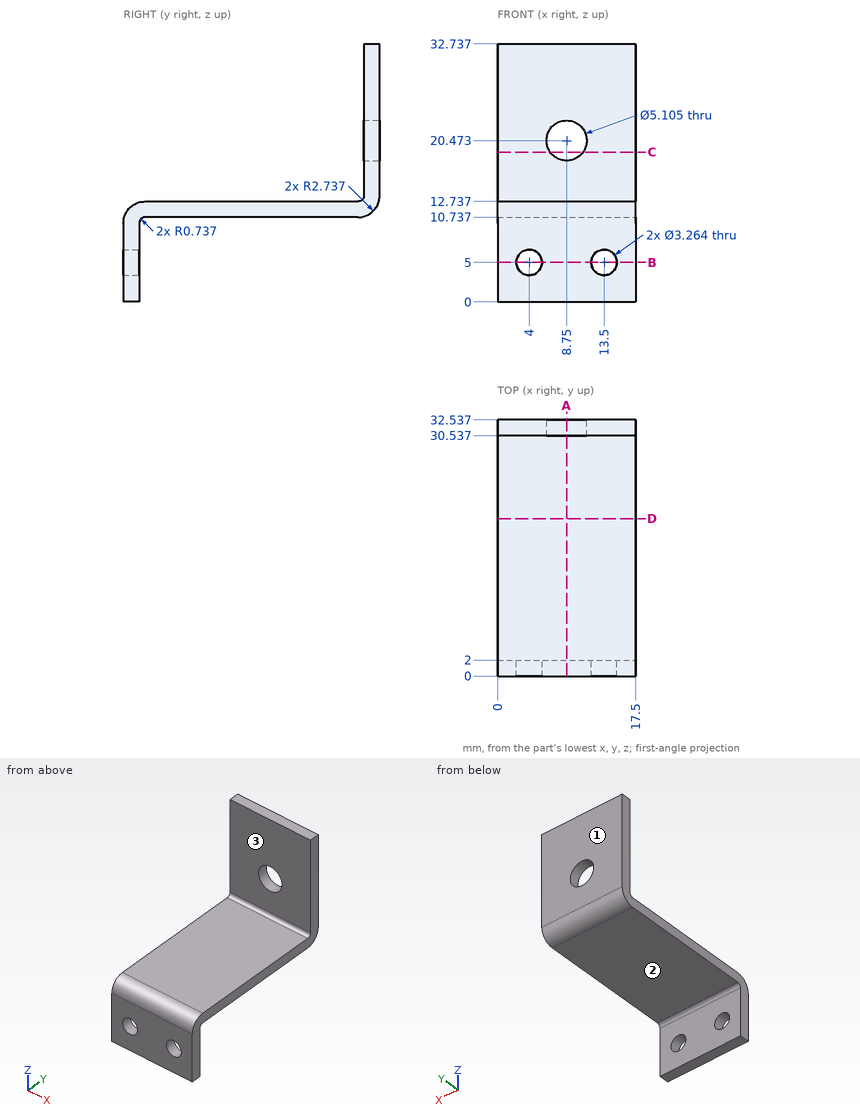
Study the drawing (mm; zero at the part's minimum x, y, z) and answer. A direction names the side the tool comes from. Coordinates: 2 decimals unless noted, no trailing zeros. Loops run counter-clockwise (first coordinate to the right, second up) from the corner with the lowest first, then second, coordinate; pieces in that order, holes last. Notation, with made-up numbers: (-32, 56.5) -> (8, 56.5) arc R23 ccw to (8, 86.5) -> close; hole circle Ø2 at (36, 11.5). An arc over 180 degrees is marked (long way). Write each question's results on one line, items separated by ' | '. Start each with the question number.
1) Find section B-B on z = 5. Determine the outline of the cut face in (x, y).
2) For the marked faces 1, 2 and 3, determine the directions among +Z, -Z, +X, -X, +Y, -Y from which every point of the face is accessible in a straight line to the end or side of a thin tool.
3) Find section D-D on y = 20. Determine the outline of the cut face in (x, z).
4) Flat-ended cylindrical pins translate along their axes: P1, Ø5, axis at x = 15.5, z = 17.5, coming from the -Y side; P2, Ø8, axis at x = 7, y = 7, coming from the +Z side; P3, Ø2, axis at x = 11.5, z = 12, coming from the -Y side; P4, Ø4, axis at x = 13.5, z = 5, coming from the -Y side. Find the tip coordinate at first contact, or state that the pin passes through.
5) Find section C-C on z = 19. Determine the outline of the cut face in (x, y) (1 decimal).
6) Consider line 1 along Y through (x, z) = (4.25, 9.5); line 2 along Y through (x, z) = (12.25, 19.5); line 3 along Z through (x, y) = (11, 5). Determine where each line is inside the solid, lowest interval first.
7) Find section A-A on x = 8.75. Determine the outline of the cut face in (y, z).
Response values:
1) outline: (0, 0) -> (2.37, 0) -> (2.37, 2) -> (0, 2) -> close; (5.63, 0) -> (11.87, 0) -> (11.87, 2) -> (5.63, 2) -> close; (15.13, 0) -> (17.5, 0) -> (17.5, 2) -> (15.13, 2) -> close
2) face 1: +Z, -Z, +X, -X, +Y | face 2: -Z, +X, -X, +Y | face 3: +Z, +X, -X, -Y
3) outline: (0, 10.74) -> (17.5, 10.74) -> (17.5, 12.74) -> (0, 12.74) -> close
4) P1: stops at y = 30.54 | P2: stops at z = 12.74 | P3: stops at y = 0.19 | P4: stops at y = 0
5) outline: (0, 30.5) -> (6.7, 30.5) -> (6.7, 32.5) -> (0, 32.5) -> close; (10.8, 30.5) -> (17.5, 30.5) -> (17.5, 32.5) -> (10.8, 32.5) -> close
6) line 1: y = 0 to 2 | line 2: y = 30.54 to 32.54 | line 3: z = 10.74 to 12.74
7) outline: (0, 0) -> (2, 0) -> (2, 10) arc R0.74 cw to (2.74, 10.74) -> (29.8, 10.74) arc R2.74 ccw to (32.54, 13.47) -> (32.54, 17.92) -> (30.54, 17.92) -> (30.54, 13.47) arc R0.74 cw to (29.8, 12.74) -> (2.74, 12.74) arc R2.74 ccw to (0, 10) -> close; (30.54, 23.03) -> (32.54, 23.03) -> (32.54, 32.74) -> (30.54, 32.74) -> close
